Here's how the part is built. I have some questions about the finished solid (model axes, mm). Face numbers are marked on the shaded views. A direction names the side the tool comes from. Round coordinates to 2 decimals unless told otherwise and drop trailing zeros. Loops run counter-clockwise (first coordinate to the right, second up) from the corner with the lowest first, then second, coordinate; pieces in that order, holes last. Notation, with made-up numbers: M 32,-28 L 73,-28 A24 ccw 73,11 Z; hole C -34,33.5 d2. An arc over 180 degrees is marked long. Answer as a JSON object with one key per item and string values.
Autodesk Fusion 360 part; units mm, degrees
ref_plane "工作平面1" through (0, 0, 0) normal (0, 0, 1) x (1, 0, 0)
sketch "草图1" plane through (0, 0, 0) normal (0, 0, 1) x (1, 0, 0)
  line L0 (-26, -22) -> (26, -22)
  line L1 (26, -22) -> (28, -20)
  line L2 (28, -20) -> (28, 20)
  line L3 (28, 20) -> (26, 22)
  line L4 (26, 22) -> (-26, 22)
  line L5 (-26, 22) -> (-28, 20)
  line L6 (-28, 20) -> (-28, -20)
  line L7 (-28, -20) -> (-26, -22)
extrude "56 x 44 x 7 platform" add sketch "草图1" along normal blind 7
ref_plane "工作平面2" through (0, 0, 7) normal (0, 0, 1) x (1, 0, 0)
sketch "草图2" plane through (0, 0, 7) normal (0, 0, 1) x (1, 0, 0)
  line L0 (-28, -22) -> (-20.49, -22)
  line L1 (-20.49, -22) -> (-20.49, 22)
  line L2 (-20.49, 22) -> (-28, 22)
  line L3 (-28, 22) -> (-28, -22)
ref_plane "工作平面3" through (0, 0, 12.2) normal (0, 0, 1) x (1, 0, 0)
sketch "草图3" plane through (0, 0, 12.2) normal (0, 0, 1) x (1, 0, 0)
  line L0 (-28, -22) -> (-16.33, -22)
  line L1 (-16.33, -22) -> (-16.33, 22)
  line L2 (-16.33, 22) -> (-28, 22)
  line L3 (-28, 22) -> (-28, -22)
loft "Dovetail retaining rail 0.8 to 1 -1" add profiles "草图2", "草图3" section 1 section 2
ref_plane "工作平面4" through (0, 0, 6.7) normal (0, 0, 1) x (1, 0, 0)
sketch "草图4" plane through (0, 0, 6.7) normal (0, 0, 1) x (1, 0, 0)
  line L0 (-23.4, -22) -> (-22.5, -22)
  line L1 (-22.5, -22) -> (-22.5, 13)
  line L2 (-22.5, 13) -> (-23.4, 13)
  line L3 (-23.4, 13) -> (-23.4, -22)
extrude "0.9 mm longitudinal flexure slot -1" cut sketch "草图4" along normal blind 5.8
ref_plane "工作平面5" through (0, 0, 6.7) normal (0, 0, 1) x (1, 0, 0)
sketch "草图5" plane through (0, 0, 6.7) normal (0, 0, 1) x (1, 0, 0)
  line L0 (-22.5, -22) -> (-15, -22)
  line L1 (-15, -22) -> (-15, 13)
  line L2 (-15, 13) -> (-22.5, 13)
  line L3 (-22.5, 13) -> (-22.5, -22)
extrude "0.8 mm flexure underside relief -1" cut sketch "草图5" along normal blind 0.8
ref_plane "工作平面6" through (0, 0, 7.6) normal (0, 0, 1) x (1, 0, 0)
sketch "草图6" plane through (0, 0, 7.6) normal (0, 0, 1) x (1, 0, 0)
  line L0 (-20.21, -6) -> (-20.21, 11)
  line L1 (-20.21, 11) -> (-19.66, 11)
  line L2 (-19.66, 11) -> (-19.66, 2)
  line L3 (-19.66, 2) -> (-20.11, -6)
  line L4 (-20.11, -6) -> (-20.21, -6)
ref_plane "工作平面7" through (0, 0, 11.8) normal (0, 0, 1) x (1, 0, 0)
sketch "草图7" plane through (0, 0, 11.8) normal (0, 0, 1) x (1, 0, 0)
  line L0 (-16.85, -6) -> (-16.85, 11)
  line L1 (-16.85, 11) -> (-16.3, 11)
  line L2 (-16.3, 11) -> (-16.3, 2)
  line L3 (-16.3, 2) -> (-16.75, -6)
  line L4 (-16.75, -6) -> (-16.85, -6)
loft "Tapered friction contact rib -1" add profiles "草图6", "草图7" section 1 section 2
ref_plane "工作平面8" through (0, 0, 7) normal (0, 0, 1) x (1, 0, 0)
sketch "草图8" plane through (0, 0, 7) normal (0, 0, 1) x (1, 0, 0)
  line L0 (20.49, -22) -> (28, -22)
  line L1 (28, -22) -> (28, 22)
  line L2 (28, 22) -> (20.49, 22)
  line L3 (20.49, 22) -> (20.49, -22)
ref_plane "工作平面9" through (0, 0, 12.2) normal (0, 0, 1) x (1, 0, 0)
sketch "草图9" plane through (0, 0, 12.2) normal (0, 0, 1) x (1, 0, 0)
  line L0 (16.33, -22) -> (28, -22)
  line L1 (28, -22) -> (28, 22)
  line L2 (28, 22) -> (16.33, 22)
  line L3 (16.33, 22) -> (16.33, -22)
loft "Dovetail retaining rail 0.8 to 1 1" add profiles "草图8", "草图9" section 1 section 2
ref_plane "工作平面10" through (0, 0, 6.7) normal (0, 0, 1) x (1, 0, 0)
sketch "草图10" plane through (0, 0, 6.7) normal (0, 0, 1) x (1, 0, 0)
  line L0 (22.5, -22) -> (23.4, -22)
  line L1 (23.4, -22) -> (23.4, 13)
  line L2 (23.4, 13) -> (22.5, 13)
  line L3 (22.5, 13) -> (22.5, -22)
extrude "0.9 mm longitudinal flexure slot 1" cut sketch "草图10" along normal blind 5.8
ref_plane "工作平面11" through (0, 0, 6.7) normal (0, 0, 1) x (1, 0, 0)
sketch "草图11" plane through (0, 0, 6.7) normal (0, 0, 1) x (1, 0, 0)
  line L0 (15, -22) -> (22.5, -22)
  line L1 (22.5, -22) -> (22.5, 13)
  line L2 (22.5, 13) -> (15, 13)
  line L3 (15, 13) -> (15, -22)
extrude "0.8 mm flexure underside relief 1" cut sketch "草图11" along normal blind 0.8
ref_plane "工作平面12" through (0, 0, 7.6) normal (0, 0, 1) x (1, 0, 0)
sketch "草图12" plane through (0, 0, 7.6) normal (0, 0, 1) x (1, 0, 0)
  line L0 (20.21, -6) -> (20.21, 11)
  line L1 (20.21, 11) -> (19.66, 11)
  line L2 (19.66, 11) -> (19.66, 2)
  line L3 (19.66, 2) -> (20.11, -6)
  line L4 (20.11, -6) -> (20.21, -6)
ref_plane "工作平面13" through (0, 0, 11.8) normal (0, 0, 1) x (1, 0, 0)
sketch "草图13" plane through (0, 0, 11.8) normal (0, 0, 1) x (1, 0, 0)
  line L0 (16.85, -6) -> (16.85, 11)
  line L1 (16.85, 11) -> (16.3, 11)
  line L2 (16.3, 11) -> (16.3, 2)
  line L3 (16.3, 2) -> (16.75, -6)
  line L4 (16.75, -6) -> (16.85, -6)
loft "Tapered friction contact rib 1" add profiles "草图12", "草图13" section 1 section 2
ref_plane "工作平面14" through (0, 0, 7) normal (0, 0, 1) x (1, 0, 0)
sketch "草图14" plane through (0, 0, 7) normal (0, 0, 1) x (1, 0, 0)
  line L0 (-16.5, 19.4) -> (16.5, 19.4)
  line L1 (16.5, 19.4) -> (16.5, 22)
  line L2 (16.5, 22) -> (-16.5, 22)
  line L3 (-16.5, 22) -> (-16.5, 19.4)
extrude "Closed insertion end stop" add sketch "草图14" along normal blind 5.2
ref_plane "工作平面15" through (0, 0, 0) normal (0, 0, 1) x (1, 0, 0)
sketch "草图15" plane through (0, 0, 0) normal (0, 0, 1) x (1, 0, 0)
  circle A0 centre (0, 0) radius 7.5
extrude "15 mm screw and driver access" cut sketch "草图15" along normal blind 7
move_body "Align camera long edge with gimbal arm - 90 degrees" bodies 1 to x (0, 1, 0) y (-1, 0, 0) z (0, 0, 1) at (0, 0, 0)
ref_plane "工作平面16" through (0, 0, 0) normal (0, 0, 1) x (1, 0, 0)
sketch "草图16" plane through (0, 0, 0) normal (0, 0, 1) x (1, 0, 0)
  line L0 (7.8, -28) -> (11.4, -28)
  line L1 (11.4, -28) -> (11.4, -21.95)
  line L2 (11.4, -21.95) -> (7.8, -21.95)
  line L3 (7.8, -21.95) -> (7.8, -28)
extrude "Clear original raised tab and root fillet" cut sketch "草图16" along normal blind 12.3
ref_plane "工作平面17" through (0, 0, 0) normal (0, 0, 1) x (1, 0, 0)
sketch "草图17" plane through (0, 0, 0) normal (0, 0, 1) x (1, 0, 0)
  line L0 (7.8, 25.95) -> (11.4, 25.95)
  line L1 (11.4, 25.95) -> (11.4, 28)
  line L2 (11.4, 28) -> (7.8, 28)
  line L3 (7.8, 28) -> (7.8, 25.95)
extrude "Clear original raised tab and root fillet (1)" cut sketch "草图17" along normal blind 12.3
ref_plane "工作平面18" through (0, 0, -2.1) normal (0, 0, 1) x (1, 0, 0)
sketch "草图18" plane through (0, 0, -2.1) normal (0, 0, 1) x (1, 0, 0)
  line L0 (-8.5, -20) -> (-6.3, -20)
  line L1 (-6.3, -20) -> (-6.3, 20)
  line L2 (-6.3, 20) -> (-8.5, 20)
  line L3 (-8.5, 20) -> (-8.5, -20)
extrude "Arm lateral locating shoulder" add sketch "草图18" along normal blind 2.1
ref_plane "工作平面19" through (0, 0, -2.1) normal (0, 0, 1) x (1, 0, 0)
sketch "草图19" plane through (0, 0, -2.1) normal (0, 0, 1) x (1, 0, 0)
  line L0 (8.3, -20) -> (10.5, -20)
  line L1 (10.5, -20) -> (10.5, 20)
  line L2 (10.5, 20) -> (8.3, 20)
  line L3 (8.3, 20) -> (8.3, -20)
extrude "Arm lateral locating shoulder (1)" add sketch "草图19" along normal blind 2.1
ref_plane "工作平面20" through (0, 0, 0) normal (0, 0, 1) x (1, 0, 0)
sketch "草图20" plane through (0, 0, 0) normal (0, 0, 1) x (1, 0, 0)
  circle A0 centre (0, -16) radius 1.2
extrude "M2 through clearance at y -16.0" cut sketch "草图20" along normal blind 7
ref_plane "工作平面21" through (0, 0, 5.3) normal (0, 0, 1) x (1, 0, 0)
sketch "草图21" plane through (0, 0, 5.3) normal (0, 0, 1) x (1, 0, 0)
  circle A0 centre (0, -16) radius 2.25
extrude "M2 head recess at y -16.0" cut sketch "草图21" along normal blind 1.7
ref_plane "工作平面22" through (0, 0, 0) normal (0, 0, 1) x (1, 0, 0)
sketch "草图22" plane through (0, 0, 0) normal (0, 0, 1) x (1, 0, 0)
  circle A0 centre (0, 16) radius 1.2
extrude "M2 through clearance at y 16.0" cut sketch "草图22" along normal blind 7
ref_plane "工作平面23" through (0, 0, 5.3) normal (0, 0, 1) x (1, 0, 0)
sketch "草图23" plane through (0, 0, 5.3) normal (0, 0, 1) x (1, 0, 0)
  circle A0 centre (0, 16) radius 2.25
extrude "M2 head recess at y 16.0" cut sketch "草图23" along normal blind 1.7
ref_plane "工作平面24" through (0, 0, 0) normal (0, 0, 1) x (1, 0, 0)
sketch "草图24" plane through (0, 0, 0) normal (0, 0, 1) x (1, 0, 0)
  line L0 (5, -32.15) -> (8.7, -32.15)
  line L1 (8.7, -32.15) -> (8.7, -24.15)
  line L2 (8.7, -24.15) -> (5, -24.15)
  line L3 (5, -24.15) -> (5, -32.15)
extrude "Ear for original 3.2 mm side hole at arm y -28.15" add sketch "草图24" along normal blind 7.2
ref_plane "工作平面25" through (0, 0, 0) normal (0, 0, 1) x (1, 0, 0)
sketch "草图25" plane through (0, 0, 0) normal (0, 0, 1) x (1, 0, 0)
  line L0 (7.8, -32.15) -> (8.9, -32.15)
  line L1 (8.9, -32.15) -> (8.9, -24.15)
  line L2 (8.9, -24.15) -> (7.8, -24.15)
  line L3 (7.8, -24.15) -> (7.8, -32.15)
extrude "Ear relief around original arm root radius" cut sketch "草图25" along normal blind 1.3
ref_plane "工作平面26" through (4.9, 0, 0) normal (1, 0, 0) x (0, 1, 0)
sketch "草图26" plane through (4.9, 0, 0) normal (1, 0, 0) x (0, 0, -1)
  circle A0 centre (-5, -28.15) radius 1.6
extrude "Side rivet ear clearance" cut sketch "草图26" along normal blind 4
ref_plane "工作平面27" through (0, 0, 0) normal (0, 0, 1) x (1, 0, 0)
sketch "草图27" plane through (0, 0, 0) normal (0, 0, 1) x (1, 0, 0)
  line L0 (5, 27.5) -> (8.7, 27.5)
  line L1 (8.7, 27.5) -> (8.7, 40.85)
  line L2 (8.7, 40.85) -> (5, 40.85)
  line L3 (5, 40.85) -> (5, 27.5)
extrude "Ear for original 3.2 mm side hole at arm y 36.85" add sketch "草图27" along normal blind 7.2
ref_plane "工作平面28" through (0, 0, 0) normal (0, 0, 1) x (1, 0, 0)
sketch "草图28" plane through (0, 0, 0) normal (0, 0, 1) x (1, 0, 0)
  line L0 (7.8, 27.5) -> (8.9, 27.5)
  line L1 (8.9, 27.5) -> (8.9, 40.85)
  line L2 (8.9, 40.85) -> (7.8, 40.85)
  line L3 (7.8, 40.85) -> (7.8, 27.5)
extrude "Ear relief around original arm root radius (1)" cut sketch "草图28" along normal blind 1.3
ref_plane "工作平面29" through (4.9, 0, 0) normal (1, 0, 0) x (0, 1, 0)
sketch "草图29" plane through (4.9, 0, 0) normal (1, 0, 0) x (0, 0, -1)
  circle A0 centre (-5, 36.85) radius 1.6
extrude "Side rivet ear clearance (1)" cut sketch "草图29" along normal blind 4
ref_plane "工作平面30" through (4.9, 0, 0) normal (1, 0, 0) x (0, 1, 0)
sketch "草图30" plane through (4.9, 0, 0) normal (1, 0, 0) x (0, 0, -1)
  circle A0 centre (-5, -28.15) radius 1.6
extrude "Side rivet full passage clearance" cut sketch "草图30" along normal blind 20
ref_plane "工作平面31" through (2.9, 0, 0) normal (1, 0, 0) x (0, 1, 0)
sketch "草图31" plane through (2.9, 0, 0) normal (1, 0, 0) x (0, 0, -1)
  circle A0 centre (-5, -28.15) radius 2.9
extrude "Side rivet flange counterbore" cut sketch "草图31" along normal blind 2.2
ref_plane "工作平面32" through (4.9, 0, 0) normal (1, 0, 0) x (0, 1, 0)
sketch "草图32" plane through (4.9, 0, 0) normal (1, 0, 0) x (0, 0, -1)
  circle A0 centre (-5, 36.85) radius 1.6
ref_plane "工作平面33" through (2.9, 0, 0) normal (1, 0, 0) x (0, 1, 0)
sketch "草图33" plane through (2.9, 0, 0) normal (1, 0, 0) x (0, 0, -1)
  circle A0 centre (-5, 36.85) radius 2.9
extrude "Side rivet flange counterbore (1)" cut sketch "草图33" along normal blind 2.2
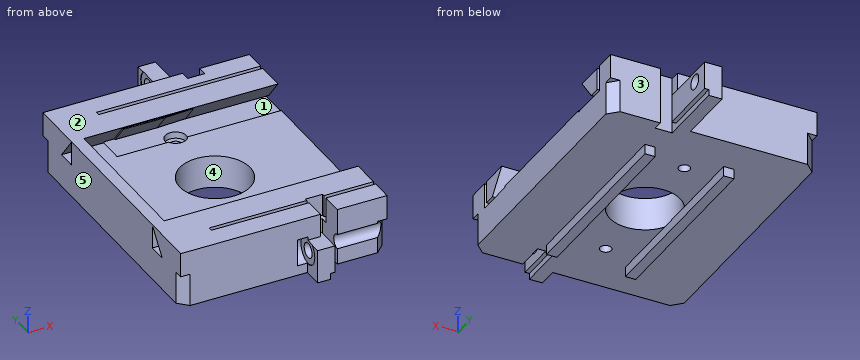
Item 1: I want a section at C-C on y = -12. List the corners of the cut face in (x, z) for me, plus the area to 3 significant figures.
Solution:
{"outline": "M -22,0 L -8.5,0 L -8.5,-2.1 L -6.3,-2.1 L -6.3,0 L 8.3,0 L 8.3,-2.1 L 10.5,-2.1 L 10.5,0 L 22,0 L 22,7 L -19.4,7 L -19.4,12.2 L -22,12.2 Z", "area": "331 mm2"}
Item 2: I want a section at B-B on y = 0. List the corners of the cut face in (x, z) for me.
Solution:
{"outline": "M -22,0 L -8.5,0 L -8.5,-2.1 L -6.3,-2.1 L -6.3,0 L -7.5,0 L -7.5,7 L -19.4,7 L -19.4,12.2 L -22,12.2 Z; M 7.5,0 L 8.3,0 L 8.3,-2.1 L 10.5,-2.1 L 10.5,0 L 22,0 L 22,7 L 7.5,7 Z"}
Item 3: I want a section at A-A on x = 6. Count the separate pieces of the cut face and the enclosed holes in it, plus the area to 3 significant figures.
Solution:
{"separate pieces": "4", "enclosed holes": "2", "area": "518 mm2"}
Item 4: For P1, Ø3, axis at x = 6, y = -29, coming from the +Z side; P2, Ø3, axis at x = -20, z = 10, coming from the -Y side; P3, Ø0.6, axis at y = 27, z = 3.5, coming from the -X side; P4, Ø8, axis at x = 15, z = 9, coming from the +Y side, each with a flat end and sliding along its axis, tell me the tip position at first contact or that it passes through.
Solution:
{"P1": "stops at z = 12.2", "P2": "stops at y = -28", "P3": "stops at x = -21.3", "P4": "stops at y = 28"}
Item 5: We'd pull the mould along X, two halves only. Please class the marked faces 3, 4 and 5: +X half, -X half, draft (parallel to the pull), parting line (faces both ways), or undercut.
Solution:
{"face 3": "draft", "face 4": "undercut", "face 5": "-X half"}
Item 6: For the marked faces 1 and 2, which set-ups out of +Z, -Z, +X, -X, +Y, -Y let a thin tool reach every point of the face, with its end or its side?
Solution:
{"face 1": "+X", "face 2": "+Z, +X, -X, +Y, -Y"}
Item 7: If I drill on L1, parallel to X at y = 16, z = 2.4; L2, parallel to X at y = 16, z = 5.9; L3, parallel to Y at x = 0, z = 6, over which ranges is the centre line in solid material (lowest first)? Write a range as from..to.
Solution:
{"L1": "x = -22..-1.2, 1.2..22", "L2": "x = -22..-2.25, 2.25..22", "L3": "y = -28..-18.25, -13.75..-7.5, 7.5..13.75, 18.25..28"}
